CAD build for the part. Positions are in the model's coordinates, mm. Coordinates: 2 decimals unless noted, no trailing zeros. Write each loop counter-clockwise with the first axis right and the second up, starting at its lowest first coordinate (ties: lowest second). Pieces come first, ordered by that corner, then holes. Notation, with made-up numbers: (84.25, -37.5) - (111.25, -37.5) arc R28 ccw to (111.25, -3.5) - close; hole circle Ø5 at (48, -14). An arc over 180 degrees is marked (long way). Answer in a Markdown table with one row per item. Add a question column.
Q1. Band-saw the part on A-A (x = 117). List the corners of the cut face in (y, z).
Q2. Pin check, flat tips, straight feed: pin 1 (10.5 mm diameter, centred on x = 117, z = -15, fed in from -Y); pin 2 (8.5 mm diameter, centred on x = 117, z = -135, fed in from -Y); pin 3 (7.5 mm diameter, centred on x = 117, z = -80, fed in from +Y). Stop position of each tip, or through.
Q3. Band-saw the part on B-B (z = -70). List the corners of the cut face in (x, y), and give its area (3 significant figures).
Q4. Drill centre lines: line 1 along X through (y, z) = (0.75, -80); line 2 along Z through (x, y) = (15, 1.45); line 3 along Z through (x, y) = (66, 1.25). Where is each one in solid material? Low to high. Write a range as from..to.
Q5. Band-saw the part on D-D (z = -135). List the corners of the cut face in (x, y).
Q6. Band-saw the part on C-C (x = 66). List the corners of the cut face in (y, z).
```python
from build123d import *

# Parameters (mm, degrees)
SKETCH1_W                                       = 132
SKETCH1_H                                       = 150
BOSS_EXTRUDE1_DEPTH                             = 5
CSK_FOR_M6_FLAT_HEAD_MACHINE_SCREW1_D           = 6.6
CSK_FOR_M6_FLAT_HEAD_MACHINE_SCREW1_DEPTH       = 10
CSK_FOR_M6_FLAT_HEAD_MACHINE_SCREW1_CSINK_D     = 12.6
CSK_FOR_M6_FLAT_HEAD_MACHINE_SCREW1_CSINK_ANGLE = 90
CSK_FOR_M6_FLAT_HEAD_MACHINE_SCREW1_TIP         = 1.982840043
CSK_FOR_M6_FLAT_HEAD_MACHINE_SCREW2_D           = 6.6
CSK_FOR_M6_FLAT_HEAD_MACHINE_SCREW2_DEPTH       = 10
CSK_FOR_M6_FLAT_HEAD_MACHINE_SCREW2_CSINK_D     = 12.6
CSK_FOR_M6_FLAT_HEAD_MACHINE_SCREW2_CSINK_ANGLE = 90
CSK_FOR_M6_FLAT_HEAD_MACHINE_SCREW2_TIP         = 1.982840043
FILLET1_R                                       = 5


with BuildPart() as part:
    # Sketch1 → Boss-Extrude1 (new body)
    with BuildSketch(Plane(origin=(0, 0, 0), x_dir=(1, 0, 0), z_dir=(0, 1, 0))):
        with Locations((66, 75)):
            Rectangle(SKETCH1_W, SKETCH1_H)
    extrude(amount=BOSS_EXTRUDE1_DEPTH)

    # CSK for M6 Flat Head Machine Screw1
    with Locations(Plane(origin=(0, 5, 0), x_dir=(1, 0, 0), z_dir=(0, 1, 0))):
        with Locations((15, 80), (66, 70), (117, 80)):
            CounterSinkHole(CSK_FOR_M6_FLAT_HEAD_MACHINE_SCREW1_D / 2, CSK_FOR_M6_FLAT_HEAD_MACHINE_SCREW1_CSINK_D / 2, depth=CSK_FOR_M6_FLAT_HEAD_MACHINE_SCREW1_DEPTH, counter_sink_angle=CSK_FOR_M6_FLAT_HEAD_MACHINE_SCREW1_CSINK_ANGLE)
            with Locations((0, 0, -(CSK_FOR_M6_FLAT_HEAD_MACHINE_SCREW1_DEPTH + CSK_FOR_M6_FLAT_HEAD_MACHINE_SCREW1_TIP / 2))):  # 118° drill point
                Cone(0, CSK_FOR_M6_FLAT_HEAD_MACHINE_SCREW1_D / 2, CSK_FOR_M6_FLAT_HEAD_MACHINE_SCREW1_TIP, mode=Mode.SUBTRACT)

    # CSK for M6 Flat Head Machine Screw2
    with Locations(Plane(origin=(0, 0, 0), x_dir=(-1, 0, 0), z_dir=(0, -1, 0))):
        with Locations((-15, 15), (-117, 15), (-117, 135), (-15, 135)):
            CounterSinkHole(CSK_FOR_M6_FLAT_HEAD_MACHINE_SCREW2_D / 2, CSK_FOR_M6_FLAT_HEAD_MACHINE_SCREW2_CSINK_D / 2, depth=CSK_FOR_M6_FLAT_HEAD_MACHINE_SCREW2_DEPTH, counter_sink_angle=CSK_FOR_M6_FLAT_HEAD_MACHINE_SCREW2_CSINK_ANGLE)
            with Locations((0, 0, -(CSK_FOR_M6_FLAT_HEAD_MACHINE_SCREW2_DEPTH + CSK_FOR_M6_FLAT_HEAD_MACHINE_SCREW2_TIP / 2))):  # 118° drill point
                Cone(0, CSK_FOR_M6_FLAT_HEAD_MACHINE_SCREW2_D / 2, CSK_FOR_M6_FLAT_HEAD_MACHINE_SCREW2_TIP, mode=Mode.SUBTRACT)

    # Fillet1
    fillet1_edges = [part.edges().sort_by_distance(p)[0] for p in [
        (0, 2.5, -150),
        (132, 2.5, -150),
        (132, 2.5, 0),
        (0, 2.5, 0),
    ]]
    fillet(fillet1_edges, radius=FILLET1_R)


solid = part.part
```
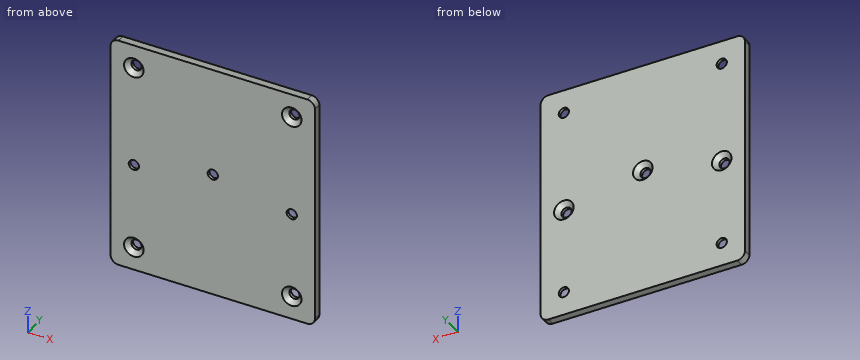
Checked values:
| question | item | result |
|---|---|---|
| 1 | outline | (0, -150) - (5, -150) - (5, -138.3) - (3, -138.3) - (0, -141.3) - close; (0, -128.7) - (3, -131.7) - (5, -131.7) - (5, -86.3) - (2, -83.3) - (0, -83.3) - close; (0, -76.7) - (2, -76.7) - (5, -73.7) - (5, -18.3) - (3, -18.3) - (0, -21.3) - close; (0, -8.7) - (3, -11.7) - (5, -11.7) - (5, 0) - (0, 0) - close |
| 2 | pin 1 | stops at y = 1.05 |
| 2 | pin 2 | stops at y = 2.05 |
| 2 | pin 3 | stops at y = 2.45 |
| 3 | outline | (0, 0) - (62.7, 0) - (62.7, 2) - (59.7, 5) - (0, 5) - close; (69.3, 0) - (132, 0) - (132, 5) - (72.3, 5) - (69.3, 2) - close |
| 3 | area | 618 mm² |
| 4 | line 1 | x = 0..11.7, 18.3..113.7, 120.3..132 |
| 4 | line 2 | z = -150..-139.85, -130.15..-83.3, -76.7..-19.85, -10.15..0 |
| 4 | line 3 | z = -150..-73.3, -66.7..0 |
| 5 | outline | (0, 0) - (8.7, 0) - (11.7, 3) - (11.7, 5) - (0, 5) - close; (18.3, 3) - (21.3, 0) - (110.7, 0) - (113.7, 3) - (113.7, 5) - (18.3, 5) - close; (120.3, 3) - (123.3, 0) - (132, 0) - (132, 5) - (120.3, 5) - close |
| 6 | outline | (0, -150) - (5, -150) - (5, -76.3) - (2, -73.3) - (0, -73.3) - close; (0, -66.7) - (2, -66.7) - (5, -63.7) - (5, 0) - (0, 0) - close |
